```python
from build123d import *

# Parameters (mm, degrees)
SKETCH2_R           = 145
SKETCH2_R_2         = 105
BOSS_EXTRUDE1_START = -40
SKETCH3_W           = 360
SKETCH3_H           = 360
SKETCH3_R           = 145
BOSS_EXTRUDE1_DEPTH = 40
SKETCH4_W           = 360
SKETCH4_H           = 360
SKETCH4_R           = 145
BOSS_EXTRUDE2_DEPTH = 40
FILLET1_R           = 20
CHAMFER1_SIZE       = 10
SKETCH5_R           = 30
CUT_EXTRUDE1_DEPTH  = 10
CUT_EXTRUDE2_REACH  = 734.735
SKETCH6_R           = 15
CIRPATTERN1_COUNT   = 4
SKETCH7_R           = 30
CUT_EXTRUDE3_DEPTH  = 10
CUT_EXTRUDE4_REACH  = 848.699
SKETCH8_R           = 15
CIRPATTERN2_COUNT   = 4


with BuildPart() as part:
    # Sweep-Thin1: sweep along a path in Sketch1
    with BuildLine(Plane.XY) as sweep_thin1_path:
        Line((0, 0), (-150, 0))
        ThreePointArc((-150, 0), (-333.847763109, 76.152236891), (-410, 260))
        Line((-410, 260), (-410, 410))
    # Sketch2 → Sweep-Thin1 (sweep)
    with BuildSketch(Plane(origin=(0, 0, 0), x_dir=(0, 0, -1), z_dir=(1, 0, 0))):
        Circle(SKETCH2_R)
        Circle(SKETCH2_R_2, mode=Mode.SUBTRACT)
    sweep(path=sweep_thin1_path.line)

    # Sketch3 → Boss-Extrude1 (add)
    with BuildSketch(Plane(origin=(0, 0, 0), x_dir=(0, 0, -1), z_dir=(1, 0, 0)).offset(BOSS_EXTRUDE1_START)):
        Rectangle(SKETCH3_W, SKETCH3_H)
        with Locations(Location((0, 0, 0), (0, 0, 270))):
            Circle(SKETCH3_R, mode=Mode.SUBTRACT)
    extrude(amount=BOSS_EXTRUDE1_DEPTH)

    # Sketch4 → Boss-Extrude2 (add)
    with BuildSketch(Plane(origin=(0, 410, 0), x_dir=(1, 0, 0), z_dir=(0, 1, 0))):
        with Locations((-410, 0)):
            Rectangle(SKETCH4_W, SKETCH4_H)
        with Locations(Location((-410, 0, 0), (0, 0, 180))):
            Circle(SKETCH4_R, mode=Mode.SUBTRACT)
    extrude(amount=-BOSS_EXTRUDE2_DEPTH)

    # Fillet1
    fillet1_edges = [part.edges().sort_by_distance(p)[0] for p in [
        (-20, 180, -180),
        (-20, -180, -180),
        (-20, -180, 180),
        (-20, 180, 180),
        (-230, 390, -180),
        (-230, 390, 180),
        (-590, 390, 180),
        (-590, 390, -180),
    ]]
    fillet(fillet1_edges, radius=FILLET1_R)

    # Chamfer1
    chamfer1_edges = [part.edges().sort_by_distance(p)[0] for p in [
        (0, 0, 105),
        (-410, 410, 105),
    ]]
    chamfer(chamfer1_edges, length=CHAMFER1_SIZE)

    # Sketch5 → Cut-Extrude1 (cut)
    with BuildSketch(Plane(origin=(0, 0, 0), x_dir=(0, 0, -1), z_dir=(1, 0, 0))):
        with Locations((-130, 130)):
            Circle(SKETCH5_R)
    cut_extrude1 = extrude(amount=-CUT_EXTRUDE1_DEPTH, mode=Mode.SUBTRACT)

    # Sketch6 → Cut-Extrude2 (cut, up to next)
    with BuildSketch(Plane(origin=(-10, 0, 0), x_dir=(0, 0, -1), z_dir=(1, 0, 0)), mode=Mode.PRIVATE) as cut_extrude2_sk1:
        with Locations((-130, 130)):
            Circle(SKETCH6_R)
    cut_extrude2_tool1 = extrude(cut_extrude2_sk1.sketch, amount=-CUT_EXTRUDE2_REACH, mode=Mode.PRIVATE) & part.part
    cut_extrude2 = cut_extrude2_tool1.solids().sort_by_distance((-10, 130, 130))[0]
    add(cut_extrude2, mode=Mode.SUBTRACT)

    # CirPattern1: Cut-Extrude1, Cut-Extrude2 ×4 about axis
    cirpattern1_axis = Axis((0, 0, 0), (1, 0, 0))
    add([cut_extrude1.rotate(cirpattern1_axis, i * 360 / CIRPATTERN1_COUNT) for i in range(1, CIRPATTERN1_COUNT)], mode=Mode.SUBTRACT)
    add([cut_extrude2.rotate(cirpattern1_axis, i * 360 / CIRPATTERN1_COUNT) for i in range(1, CIRPATTERN1_COUNT)], mode=Mode.SUBTRACT)

    # Sketch7 → Cut-Extrude3 (cut)
    with BuildSketch(Plane(origin=(0, 410, 0), x_dir=(1, 0, 0), z_dir=(0, 1, 0))):
        with Locations(Location((-540, 130, 0), (0, 0, 180))):
            Circle(SKETCH7_R)
    cut_extrude3 = extrude(amount=-CUT_EXTRUDE3_DEPTH, mode=Mode.SUBTRACT)

    # Sketch8 → Cut-Extrude4 (cut, up to next)
    with BuildSketch(Plane(origin=(0, 400, 0), x_dir=(1, 0, 0), z_dir=(0, 1, 0)), mode=Mode.PRIVATE) as cut_extrude4_sk1:
        with Locations(Location((-540, 130, 0), (0, 0, 180))):
            Circle(SKETCH8_R)
    cut_extrude4_tool1 = extrude(cut_extrude4_sk1.sketch, amount=-CUT_EXTRUDE4_REACH, mode=Mode.PRIVATE) & part.part
    cut_extrude4 = cut_extrude4_tool1.solids().sort_by_distance((-540, 400, -130))[0]
    add(cut_extrude4, mode=Mode.SUBTRACT)

    # CirPattern2: Cut-Extrude3, Cut-Extrude4 ×4 about axis
    cirpattern2_axis = Axis((-410, 0, 0), (0, 1, 0))
    add([cut_extrude3.rotate(cirpattern2_axis, i * 360 / CIRPATTERN2_COUNT) for i in range(1, CIRPATTERN2_COUNT)], mode=Mode.SUBTRACT)
    add([cut_extrude4.rotate(cirpattern2_axis, i * 360 / CIRPATTERN2_COUNT) for i in range(1, CIRPATTERN2_COUNT)], mode=Mode.SUBTRACT)


solid = part.part
```
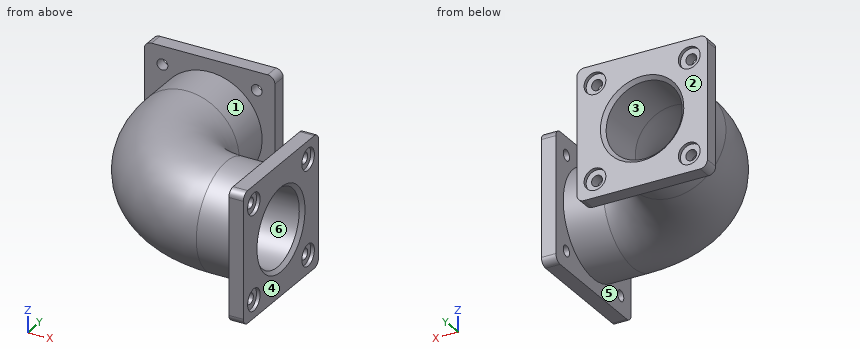
The listing builds one solid part. Answer for the finished solid, in the listing's coordinates (mm). Face numbers are marked on the shaded views. A direction names the side the tool comes from. Coordinates: 2 decimals unless noted, no trailing zeros. Loops run counter-clockwise (first coordinate to the right, second up) from the corner with the lowest first, then second, coordinate; pieces in that order, holes last. Notation, with made-up numbers: (-31.75, -25.5) -> (-15.75, -25.5) arc R27 cw to (-15.75, 6.5) -> close; hole circle Ø5 at (34, 76.5). An arc over 180 degrees is marked (long way). Return JSON: item names as keys, results as strings. Group by question number.
(1) A cutting plane is placed at D-D on x = -93. Write down the section's boundary in (y, z), and give its area (3 significant figures).
(2) A cutting plane is placed at A-A on x = -280. Count the separate pieces of the cut face and the enclosed holes in it, and give its area (3 significant figures).
(3) Determine the mould class of the marked faces 4, 5 and 6 for opening direction X: released by +X, released by -X, zero draft, split by the parting line, or undercut.
(4) Given pin 1 Ø10 at (x, y) = (-253, 181) entering from -Z; pin 2 Ø5 at (x, z) = (-92, -50.5) entering from +Y; pin 3 Ø2 at (y, z) = (310, 13) entering from -X; pin 4 Ø18 at (x, z) = (-540, -130) entering from +Y, each flat-ended and moving along its own axis, determine where each tip first touches the part or whether it passes through.
(5) Which of the six approach directions +Z, -Z, +X, -X, +Y, -Y give full straight-line access (tool end or side, diameter ignored) to the marked faces 1, 2 and 3?
(6) Find the intervals of material crossed by probe 1 along Y at (x, z) = (-7.5, -130); probe 2 along X at (y, z) = (361, 0); probe 3 along X at (y, z) = (392.5, -130), in increasing order. Write a range as from..to.
The answers:
{
 "1": {"outline": "circle Ø290 at (0, 0); hole circle Ø210 at (0, 0)", "area": "31,400 mm^2"},
 "2": {"separate pieces": "3", "enclosed holes": "1", "area": "69,900 mm^2"},
 "3": {"face 4": "released by +X", "face 5": "undercut", "face 6": "zero draft"},
 "4": {"pin 1": "stops at z = -73.16", "pin 2": "stops at y = 136.82", "pin 3": "stops at x = -554.5", "pin 4": "passes through"},
 "5": {"face 1": "none", "face 2": "+Z, -Z, +X, -X, +Y", "face 3": "+Y"},
 "6": {"probe 1": "y = -180..-160, -100..100, 160..180", "probe 2": "x = -555..-515, -305..-265", "probe 3": "x = -590..-555, -525..-295, -265..-230"}
}
